Drawing for the job (mm, zero at the part's lowest x, y, z). Round coordinates to 2 decimals unless told otherwise and drop trailing zeros. Loops run counter-clockwise (first coordinate to the right, second up) from the corner with the lowest first, then second, coordinate; pieces in that order, holes last. Notation, with made-up numbers: (39.5, 54) -> (49.5, 54) arc R18 ccw to (49.5, 83) -> close; hole circle Ø2 at (58.5, 21.25). An arc over 180 degrees is marked (long way). Put each result on its own line as item: value. Start each with the question number.
Item 1: Drill centre lines: probe 1 along Y at (x, z) = (5, 3.25); probe 2 along Y at (x, z) = (5, 6.25); probe 3 along Z at (x, y) = (4, 12.5). Where is each one in solid material? Low to high. Write a range as [from, to].
Item 2: Cut at A-A, the plane z = 5.75. List the corners of the cut face in (x, y), plus the area to 3 significant figures.
Item 3: Pull direction Y, two halves, no side cores. Call the marked faces 1, 2, 3 and 4: +Y half, -Y half, draft (parallel to the pull), parting line (faces both ways), or undercut.
Item 4: Flat gauge pins, fed straight in: pin 1 Ø4 at (x, y) = (5, 4.5) entering from +Z; pin 2 Ø3 at (x, y) = (3.5, 30) entering from +Z. Where does each tip first touch, or does it go through?
Item 5: Cut at C-C, the plane x = 5. List the corners of the cut face in (y, z), plus the area to 3 significant figures.
Item 6: Cut at B-B, the plane y = 45.5. List the corners of the cut face in (x, z), plus the area to 3 significant figures.
Item 7: Cut at D-D, the plane z = 1. List the corners of the cut face in (x, y), plus the area to 3 significant figures.
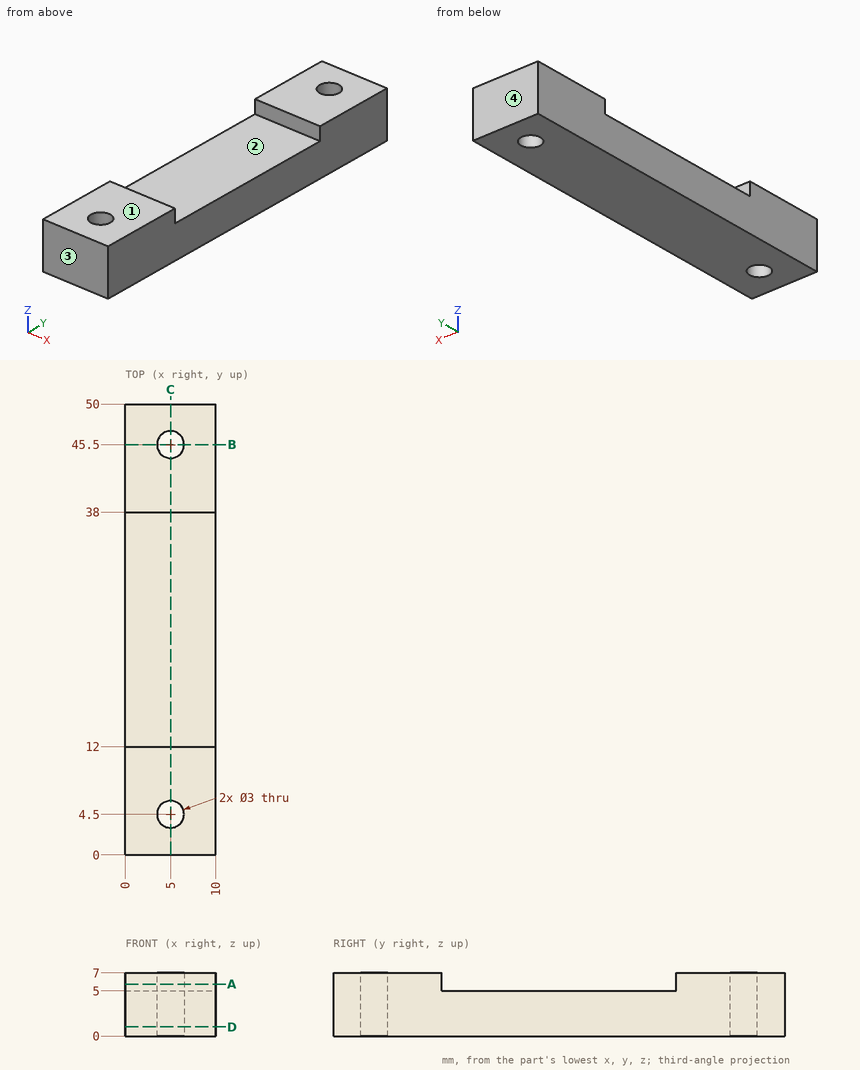
Reply:
1. probe 1: y = [0, 3], [6, 44], [47, 50]
1. probe 2: y = [0, 3], [6, 12], [38, 44], [47, 50]
1. probe 3: z = [0, 5]
2. outline: (0, 0) -> (10, 0) -> (10, 12) -> (0, 12) -> close; (0, 38) -> (10, 38) -> (10, 50) -> (0, 50) -> close; hole circle Ø3 at (5, 4.5); hole circle Ø3 at (5, 45.5)
2. area: 226 mm^2
3. face 1: draft
3. face 2: undercut
3. face 3: -Y half
3. face 4: +Y half
4. pin 1: stops at z = 7
4. pin 2: stops at z = 5
5. outline: (0, 0) -> (3, 0) -> (3, 7) -> (0, 7) -> close; (6, 0) -> (44, 0) -> (44, 7) -> (38, 7) -> (38, 5) -> (12, 5) -> (12, 7) -> (6, 7) -> close; (47, 0) -> (50, 0) -> (50, 7) -> (47, 7) -> close
5. area: 256 mm^2
6. outline: (0, 0) -> (3.5, 0) -> (3.5, 7) -> (0, 7) -> close; (6.5, 0) -> (10, 0) -> (10, 7) -> (6.5, 7) -> close
6. area: 49.0 mm^2
7. outline: (0, 0) -> (10, 0) -> (10, 50) -> (0, 50) -> close; hole circle Ø3 at (5, 4.5); hole circle Ø3 at (5, 45.5)
7. area: 486 mm^2
